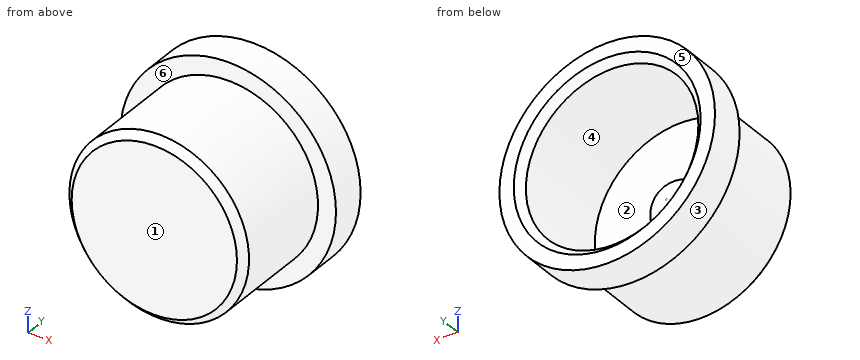
Autodesk Inventor part; units mm, degrees
ref_plane "YZ Plane" through (0, 0, 0) normal (1, 0, 0) x (0, 1, 0)
ref_plane "XZ Plane" through (0, 0, 0) normal (0, 1, 0) x (-1, 0, 0)
ref_plane "XY Plane" through (0, 0, 0) normal (0, 0, 1) x (1, 0, 0)
sketch "Szkic1" plane through (0, 0, 0) normal (0, 1, 0) x (-1, 0, 0)
  circle A0 centre (0, 0) radius 15
  circle A1 centre (0, 0) radius 12
  circle A2 centre (0, 0) radius 12.5
  circle A3 centre (0, 0) radius 4
  dimension "d0" = 30
  dimension "d1" = 24
  dimension "d2" = 25
  dimension "d12" = 8
extrude "Wyciągnięcie proste1" add sketch "Szkic1" along normal blind 20 contours A0 | A1 | A2 | A3
extrude "Wyciągnięcie proste2" cut sketch "Szkic1" against normal blind 15 from surface at 20 contours A1 | A3
extrude "Wyciągnięcie proste3" cut sketch "Szkic1" along normal blind 15 contours A0
chamfer "Faza1" distance 1 angle 45 2 edges at (12.5, 0, 0) (12, 20, 0)
extrude "Wyciągnięcie proste4" add sketch "Szkic1" along normal blind 8 contours A3
fillet "Zaokrąglenie1" radius 4 1 edges at (4, 8, 0)
properties part number "Z_screw_lower_end" material "Tworzywo sztuczne ABS"
Geometry check sheet. Reference: the model listing, model coordinates, mm. Face numbers are marked on the shaded views. A direction names the side the tool comes from. Coordinates: 2 decimals unless noted, no trailing zeros. Loops run counter-clockwise (first coordinate to the right, second up) from the corner with the lowest first, then second, coordinate; pieces in that order, holes last.
Item 1: Sectioned sample at A-A, the plane y = 10.25. Record the boundary of the cut face in (x, z).
Item 2: Sectioned sample at B-B, the plane y = 4.5. Record the boundary of the cut face in (x, z), then the cut area to 3 significant figures.
Item 3: Access from +Z, -Z, +X, -X, +Y, -Y to the whole of each face (thin tool, end or side, straight path). Record for the marked faces 5 and 6.
Item 4: Go/stop test with flat-tipped pins: pin 1 Ø1 at (x, y) = (-6, 16) entering from +Z; pin 2 Ø6 at (y, z) = (14.5, -7) entering from -X; pin 3 Ø3 at (y, z) = (10.5, 5) entering from -X. Record where each tip stops, or that it passes through.
Item 5: Thickness scan on line 1 (Z direction, x = 0, y = 11.5); line 2 (Z direction, x = 0, y = 15.75); line 3 (Y direction, x = -7.5, z = -1.5). Record the ranges inside material, lowest first.
Item 6: Release check for a two-part mould opening along X. For the marked faces 1, 2, 3 and 4 record: released by +X, released by -X, zero draft, split by the parting line, or undercut.
Check result:
1. outline: circle Ø25 at (0, 0); hole circle Ø24 at (0, 0)
2. outline: circle Ø25 at (0, 0)
2. area: 491 mm2
3. face 5: +Z, -Z, +X, -X, +Y
3. face 6: -Y
4. pin 1: stops at z = 13.96
4. pin 2: stops at x = -14.45
4. pin 3: stops at x = -12
5. line 1: z = -12.5 to -12, 12 to 12.5
5. line 2: z = -15 to -12, 12 to 15
5. line 3: y = 0 to 5
6. face 1: zero draft
6. face 2: undercut
6. face 3: split by the parting line
6. face 4: undercut
